Autodesk Inventor part; units mm, degrees
ref_plane "Work Plane1" through (1.525, 0, 0) normal (0, 0, 1) x (1, 0, 0)
ref_plane "YZ Plane" through (0, 0, 0) normal (1, 0, 0) x (0, 1, 0)
ref_plane "XZ Plane" through (0, 0, 0) normal (0, 1, 0) x (-1, 0, 0)
sketch "Sketch1" plane through (0, 0, 0) normal (0, 0, 1) x (1, 0, 0)
  line L0 (0, 9.82) -> (0, 7)
  line L1 (56, 7) -> (90, 7)
  line L2 (90, 7) -> (90, 0)
  line L3 (90, 0) -> (-0.6001, 0)
  line L4 (-18.7201, 0) -> (108.12, 0)
  line L5 (-0.6001, 0) -> (-0.6001, 9.82)
  line L6 (-0.6001, 9.82) -> (0, 9.82)
  line L7 (56, 7) -> (54.773, 7)
  line L8 (54.773, 7) -> (0, 7)
  line L9 (0, -1.964) -> (0, 11.784)
  dimension "d0" = 90
  dimension "d1" = 34
  dimension "d2" = 14
  dimension "d9" = 0.6001
  dimension "d10" = 19.64
  dimension "d13" = 1.227
  dimension "d14" = 14
revolve "Body" add sketch "Sketch1" angle 360 about axis through (90, 0, 0) along (-1, 0, 0)
sketch "Sketch2" plane through (-0.6001, 0, 0) normal (-1, 0, 0) x (0, 0, 1)
  line L0 (0, 12.1244) -> (10.5, 6.0622)
  line L1 (10.5, 6.0622) -> (10.5, -6.0622)
  line L2 (10.5, -6.0622) -> (0, -12.1244)
  line L3 (0, -12.1244) -> (-10.5, -6.0622)
  line L4 (-10.5, -6.0622) -> (-10.5, 6.0622)
  line L5 (-10.5, 6.0622) -> (0, 12.1244)
  point P0 (0, 0)
  point P1 (0, 0)
  dimension "d11" = 21
extrude "Head" add sketch "Sketch2" along normal blind 8.2
sketch "Sketch4" plane through (0, 0, 0) normal (0, 0, 1) x (1, 0, 0)
  line L0 (-8.8001, 10.5) -> (-8.8001, 12.1244)
  line L1 (-8.8001, 12.1244) -> (-7.8623, 12.1244)
  line L2 (-7.8623, 12.1244) -> (-8.8001, 10.5)
  line L3 (-10.4401, 0) -> (1.0399, 0)
  line L4 (-0.6001, 12.1244) -> (-8.8001, 12.1244)
  line L5 (-8.8001, 6.0622) -> (-8.8001, 12.1244)
  dimension "d5" = 30
  dimension "d19" = 21
revolve "Chamfer1" cut sketch "Sketch4" angle 360 about axis through (-10, 0, 0) along (1, 0, 0)
thread "Thread"
chamfer "Chamfer2" distance 1.2269 distance2 1.227 1 edges at (90, -7, 0) measured on face at (90, -1.3255, -1.9203)
ref_plane "Work Plane1" through (1.525, 0, 0) normal (0, 0, 1) x (1, 0, 0)
equation "\"d11\" = SW"
equation "\"d3\" = KOH - SD"
equation "\"d15\" = GEL"
equation "\"d6\" = -0.5 * SPD + 0.5 * GD"
equation "\"d0\" = NLG"
equation "\"d1\" = GEL"
equation "\"d2\" = GD"
equation "\"d10\" = SD2"
equation "\"d14\" = BDM"
equation "\"d5\" = ANG1"
equation "\"d19\" = SW0"
equation "\"NLG\" = 90"
equation "\"GD\" = NND"
equation "\"BDM\" = NND"
equation "\"KOH\" = 8.8"
equation "\"GEL\" = 34"
equation "\"SW\" = 21"
equation "\"SW0\" = SW"
equation "\"SPD\" = NND - 1.2269 * PTC"
equation "\"SD2\" = 19.64"
equation "\"SD\" = 0.6"
equation "\"ANG1\" = 30deg"
equation "\"GAL\" = 0.61345 * PTC"
equation "\"GUL\" = 0.61345 * PTC"
equation "\"RR\" = 0.6"
equation "\"GD1\" = THREADDIA - 1.2269 * PTC"
equation "\"THREADDIA\" = 14"
equation "\"SDH\" = SD2"
equation "\"TOA\" = 30deg"
equation "\"PTC\" = 2"
equation "\"NND\" = 14"
equation "\"E0\" = 1.155 * SW"
properties part number "ISO 4014 - M14 x 90" material "Stainless Steel, 440C"
Source: CAD feature listing. Evaluate the final solid. Frame: model axes, mm. A direction names the side the tool comes from. Give positions to 0.01 mm unless a question says otherwise; leave off trailing zeros. Order: outer loops, then holes, each group sorted by start corner. A loop starts at its lowest first (then second) coordinate and runs counter-clockwise, first axis right, second up.
(1) Contact query for flat-ended pins moving along their axis: P1, Ø1.5, axis at x = 11, z = -5.5, coming from the +Y side; P2, Ø8, axis at x = 15, y = 9.5, coming from the +Z side; P3, Ø8, axis at x = 75.5, z = 2.5, coming from the +Y side. Output: stop coordinate, or through.
(2) Material intervals for line 1 along X through (y, z) = (4, -7.5); line 2 along Z through (x, y) = (36, -3.5); line 3 along X through (y, z) = (10.25, 1.75), sorted ascending.
(3) Access query for faces 1 (the face through (-0.3, -9.81, 0.43)), 2 (the face through (-4.643, 9.051, -5.324)). Directions: +Z, -Z, +X, -X, +Y, -Y. A direction counts if a zero-diameter tool reaches every point of the face in a straight line with its end or side. Return the directions, or none.
(4) Section query A-A (x = 61). Return the cut outline in (y, z).
Outcome:
1. P1: stops at y = 5.14
1. P2: stops at z = 4.33
1. P3: stops at y = 7
2. line 1: x = -8.8 to 0
2. line 2: z = -6.06 to 6.06
2. line 3: x = -8.8 to -0.6
3. face 1: +X
3. face 2: -Z, +X, -X, +Y
4. outline: circle Ø14 at (0, 0)
